Geometry check sheet. Reference: drawing and pictorial views, mm from the part's lowest x, y, z. A direction names the side the tool comes from. Round coordinates to 2 decimals unless told otherwise and drop trailing zeros. Order: outer loops, then holes, each group sorted by start corner. A loop starts at its lowest first (then second) coordinate and runs counter-clockwise, first axis right, second up.
(1) Tool access check on the marked faces 1 and 2. Record the directions out of +Z, -Z, +X, -X, +Y, -Y that give a thin tool (end or side, any length) a straight path to the whole face; none if there is none.
(2) Thickness scan on probe 1 along Z at (x, y) = (7.75, 8.7); probe 2 along Y at (x, z) = (8.75, 2.75); probe 3 along Y at (x, z) = (12.25, 9.5). Record the ranges inside material, lowest first.
(3) Depth check by flat-ended pin: pin 1 (6 mm diameter, centred on x = 2.5, y = 12, fed in from -Z); pin 2 (2 mm diameter, centred on y = 22, z = 5.5, fed in from -X); pin 3 (4 mm diameter, centred on y = 35.5, z = 10.5, fed in from +X). Enter the tip coordinate at first touch or a pass-through.
(4) Sectioned sample at C-C, the plane z = 2.75. Enter the section's corners in (x, y).
(5) Sectioned sample at A-A, the plane y = 8.7. Enter the section's corners in (x, z), and give its area (3 significant figures).
(6) Sectioned sample at B-B, the plane y = 22. Enter the section's corners in (x, z).
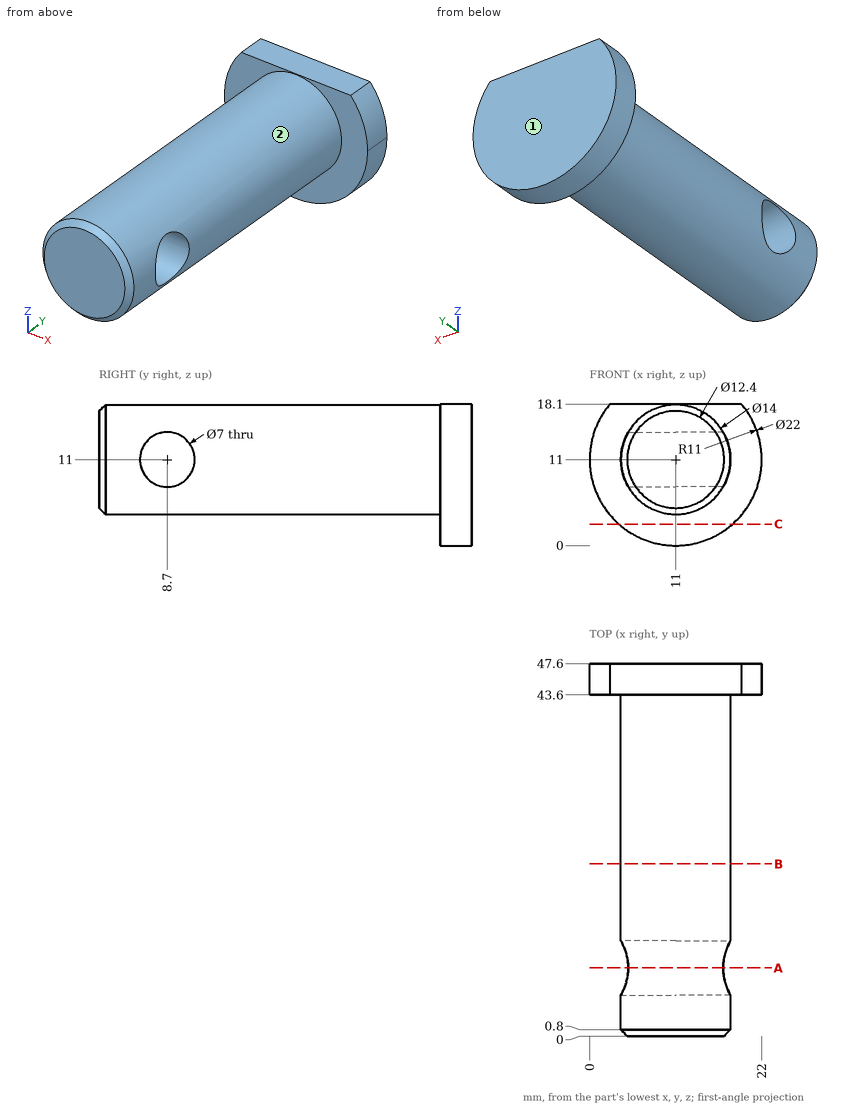
Derived:
1. face 1: +Z, -Z, +X, -X, +Y
1. face 2: -Y
2. probe 1: z = 4.8 to 7.5, 14.5 to 17.2
2. probe 2: y = 43.6 to 47.6
2. probe 3: y = 0 to 5.54, 11.86 to 47.6
3. pin 1: stops at z = 6.67
3. pin 2: stops at x = 5.64
3. pin 3: stops at x = 18
4. outline: (3.72, 43.6) - (18.28, 43.6) - (18.28, 47.6) - (3.72, 47.6) - close
5. outline: (4.94, 7.5) arc R7 ccw to (17.06, 7.5) - close; (4.94, 14.5) - (17.06, 14.5) arc R7 ccw to start
5. area: 60.2 mm2
6. outline: circle Ø14 at (11, 11)
